Geometry check sheet. Reference: the model listing, model coordinates, mm. A direction names the side the tool comes from. Give positions to 0.01 mm unless a question says otherwise; leave off trailing zeros. Order: outer loops, then holes, each group sorted by start corner. A loop starts at its lowest first (then second) coordinate and runs counter-clockwise, first axis right, second up. Notation, with made-up numbers: M 33.5,75.25 L 80.5,75.25 A18 ccw 80.5,85.25 Z; hole C 69,-6.75 d6. An arc over 180 degrees is marked long. Answer as CSV lines item,"result".
Autodesk Inventor part; units mm, degrees
ref_plane "YZ Plane" through (0, 0, 0) normal (1, 0, 0) x (0, 1, 0)
ref_plane "XZ Plane" through (0, 0, 0) normal (0, 1, 0) x (-1, 0, 0)
ref_plane "XY Plane" through (0, 0, 0) normal (0, 0, 1) x (1, 0, 0)
sketch "Sketch1" plane through (0, 0, 0) normal (0, 1, 0) x (-1, 0, 0)
  line L0 (0, 0) -> (38.1, 0)
  line L1 (38.1, 0) -> (38.1, -17)
  line L2 (38.1, -17) -> (0, -17)
  line L3 (0, -17) -> (0, 0)
  circle A0 centre (33.1, -2.5019) radius 1
  circle A1 centre (20.1, -2.5019) radius 1
  circle A2 centre (33.1, -14.5019) radius 1
  circle A3 centre (20.1, -14.5019) radius 1
  dimension "d0" = 38.1
  dimension "d1" = 17
  dimension "d41" = 2
  dimension "d42" = 2
  dimension "d43" = 2
  dimension "d44" = 2
  dimension "d45" = 13
  dimension "d46" = 12
  dimension "d47" = 2.5019
  dimension "d48" = 5
extrude "Extrusion1" add sketch "Sketch1" along normal blind 5 contours L0 L1 L2 L3 | A0 | A1 | A2 | A3
sketch "Sketch2" plane through (-38.1, 0, 0) normal (0, 0, 1) x (1, 0, 0)
  line L0 (0, 0) -> (38.1, 0)
  line L1 (38.1, 0) -> (38.1, 5)
  line L2 (0, 5) -> (38.1, 5)
  line L3 (0, 0) -> (0, 5)
  line L4 (38.1, 5) -> (25.4, 5)
  line L5 (25.4, 5) -> (25.4, 17.7)
  line L6 (25.4, 17.7) -> (38.1, 17.7)
  line L7 (38.1, 17.7) -> (38.1, 5)
  line L8 (31.75, 17.7) -> (31.75, 5) construction
  circle A0 centre (31.75, 11.35) radius 1.5
  point P0 (25.4, 5)
  dimension "d6" = 12.7
  dimension "d7" = 12.7
  dimension "d14" = 3
extrude "Extrusion2" add sketch "Sketch2" against normal up to surface (17 mm away) contours L2 L5 L6 L7 | A0
sketch "Sketch3" plane through (-12.7, 17.7, 0) normal (0, 1, 0) x (1, 0, 0)
  line L0 (12.7, 17) -> (0, 17)
  line L1 (0, 0) -> (0, 17)
  line L2 (12.7, 0) -> (0, 0)
  line L3 (12.7, 0) -> (12.7, 17)
  line L4 (0, 8.5) -> (12.7, 8.5) construction
  line L5 (0, 5.85) -> (12.7, 5.85)
  line L6 (12.7, 5.85) -> (12.7, 11.15)
  line L7 (12.7, 11.15) -> (0, 11.15)
  line L8 (0, 11.15) -> (0, 5.85)
  line L9 (0, 5.85) -> (12.7, 11.15) construction
  line L10 (12.7, 5.85) -> (0, 11.15) construction
  point P0 (12.7, 0)
  point P1 (6.35, 8.5)
  point P2 (0, 11.15)
  point P3 (0, 5.85)
  point P4 (12.7, 5.85)
  dimension "d10" = 5.3
extrude "Extrusion3" cut sketch "Sketch3" against normal up to surface (12.7 mm away) contours L3 L5 L1 L7
hole "Hole1" at (-33.1, 0, -2.5019) at (-20.1, 0, -2.5019) at (-20.1, 0, -14.5019) at (-33.1, 0, -14.5019) direction (0, 1, 0) diameter 2.5908 end through all
fillet "Fillet1" radius 6.35 4 edges at (-12.7, 17.7, -2.925) (0, 17.7, -2.925) (0, 17.7, -14.075) (-12.7, 17.7, -14.075)
chamfer "Chamfer1" distance 0.508 angle 45 9 edges at (-25.4, 5, 0) (-12.7, 8.175, 0) (-10.8402, 15.8402, 0) (0, 5.6751, 0) (-1.8598, 15.8402, -17) (-12.7, 8.175, -17) (0, 5.6751, -17) (-25.4, 5, -17) (-38.1, 5, -8.5)
hole "Hole2" at (-6.35, 11.35, 0) direction (0, 0, -1) diameter 3.6068 end through all
hole "Hole3" at (-6.35, 11.35, 0) direction (0, 0, -1) diameter 4.8006 depth 5.85
(1) Tool access check on faces 4 (the face through (-6.4, 8.6, -5.85)), 5 (the face through (-8.73, 11.66, -2.97)), 6 (the face through (-12.7, 8, -3)). Record the directions out of +Z, -Z, +X, -X, +Y, -Y that give a thin tool (end or side, any length) a straight path to the whole face; none if there is none.
The answers:
face 4,"+X, -X, +Y"
face 5,"+Z"
face 6,"+Z, -Z, -X, +Y"
(2) Section check D-D on z = -8. Enter the section's corners in (x, y).
The answers:
outline,"M -38.1,0 L 0,0 L 0,5 L -37.59,5 L -38.1,4.49 Z"
(3) Gauge pin test, flat ends, axial feed: P1, Ø8, axis at y = 14, z = -2, coming from the -X side; P2, Ø2, axis at x = -22, z = -3, coming from the +Y side; P3, Ø8, axis at x = -11, z = -11, coming from the +Y side. Record the tip position at first contact, or that the pin passes through.
The answers:
P1,"stops at x = -12.7"
P2,"stops at y = 5"
P3,"stops at y = 17.67"
(4) Draft check along Z on faces 1 (the face through (-5.25, 12.78, -14.12)), 2 (the face through (-10.63, 15.536, -0.145)), 3 (the face through (-33.98, 2.54, -1.55)). Enter one of: +Z half, -Z half, draft (parallel to the pull), parting line (faces both ways), or undercut.
The answers:
face 1,"draft"
face 2,"+Z half"
face 3,"undercut"
(5) Section check A-A on x = -20.1. Enter the section's corners in (y, z).
The answers:
outline,"M 0,-17 L 4.49,-17 L 5,-16.49 L 5,-15.8 L 0,-15.8 Z; M 0,-13.21 L 5,-13.21 L 5,-3.8 L 0,-3.8 Z; M 0,-1.21 L 5,-1.21 L 5,-0.51 L 4.49,0 L 0,0 Z"
(6) Section check B-B on y = 6. Enter the section's corners in (x, z), then the cut area to 3 significant figures.
The answers:
outline,"M -12.7,-16.49 L -12.19,-17 L -0.51,-17 L 0,-16.49 L 0,-11.15 L -12.7,-11.15 Z; M -12.7,-5.85 L 0,-5.85 L 0,-0.51 L -0.51,0 L -12.19,0 L -12.7,-0.51 Z"
area,"148 mm2"
(7) Section check C-C on z = -2. State how many separate pieces and enclosed holes the cut face has, then the cut area to 3 significant figures.
The answers:
separate pieces,"3"
enclosed holes,"1"
area,"292 mm2"
(8) Material ranges on line 1 (Z direction, x = -33.1, y = 3.25); line 2 (X direction, y = 4.5, z = -3.25); line 3 (Z direction, x = -3, y = 8.75), recorded low to high.
The answers:
line 1,"z = -17 to -15.8, -13.21 to -3.8, -1.21 to 0"
line 2,"x = -38.09 to -34.16, -32.04 to -21.16, -19.04 to 0"
line 3,"z = -17 to -11.15, -5.85 to 0"
